```python
from build123d import *

# Parameters (mm, degrees)
F0_W           = 21.1
F0_H           = 25.1
F1_DEPTH       = 62.25
F2_W           = 21.1
F2_H           = 58.25
F3_DEPTH       = 25.4
F3_DEPTH_BACK  = 25.4
F4_W           = 3
F4_H           = 2
F5_DEPTH       = 25.4
F5_DEPTH_BACK  = 25.4
F6_W           = 25.1
F6_H           = 20
F7_DEPTH       = 11.1
F8_W           = 1
F8_H           = 3
F9_DEPTH       = 25.4
F9_DEPTH_BACK  = 25.4
F10_W          = 1
F10_H          = 3
F11_DEPTH      = 25.4
F11_DEPTH_BACK = 25.4


with BuildPart() as f1:
    # F0 (on Top) → F1 (new body)
    with BuildSketch(Plane.XY):
        with Locations((0.971473, 0)):
            Rectangle(F0_W, F0_H)
    extrude(amount=F1_DEPTH)

    # F2 (on face) → F3 (cut, two sides)
    with BuildSketch(Plane.YZ.offset(11.521473)) as f3_sk:
        with Locations((0, 31.125)):
            Rectangle(F2_W, F2_H)
    extrude(amount=-F3_DEPTH, mode=Mode.SUBTRACT)
    extrude(f3_sk.sketch, amount=-F3_DEPTH_BACK, mode=Mode.SUBTRACT)

    # F4 (on face) → F5 (cut, two sides)
    with BuildSketch(Plane.YZ.offset(11.521473)) as f5_sk:
        with Locations((0, 2)):
            Rectangle(F4_W, F4_H)
    extrude(amount=-F5_DEPTH, mode=Mode.SUBTRACT)
    extrude(f5_sk.sketch, amount=-F5_DEPTH_BACK, mode=Mode.SUBTRACT)

    # F6 (on face) → F7 (cut)
    with BuildSketch(Plane.YZ.offset(11.521473)):
        with Locations((0, 31.125)):
            Rectangle(F6_W, F6_H)
    extrude(amount=-F7_DEPTH, mode=Mode.SUBTRACT)

    # F8 (on face) → F9 (cut, two sides)
    with BuildSketch(Plane(origin=(0, 0, 0), x_dir=(1, 0, 0), z_dir=(0, 0, -1))) as f9_sk:
        with Locations((-9.078527, 0)):
            Rectangle(F8_W, F8_H)
    extrude(amount=-F9_DEPTH, mode=Mode.SUBTRACT)
    extrude(f9_sk.sketch, amount=-F9_DEPTH_BACK, mode=Mode.SUBTRACT)

    # F10 (on face) → F11 (cut, two sides)
    with BuildSketch(Plane(origin=(0, 0, 60.25), x_dir=(1, 0, 0), z_dir=(0, 0, -1))) as f11_sk:
        with Locations((-9.078527, 0)):
            Rectangle(F10_W, F10_H)
    extrude(amount=-F11_DEPTH, mode=Mode.SUBTRACT)
    extrude(f11_sk.sketch, amount=-F11_DEPTH_BACK, mode=Mode.SUBTRACT)


with BuildPart() as f12_1:
    # F12: copy of F1
    add(f1.part)


solid = f1.part
```
Can you work these out from the model? Positions are in its coordinate system, mm. A direction names the side the tool comes from. Coordinates: 2 decimals unless noted, no trailing zeros. Order: outer loops, then holes, each group sorted by start corner. A loop starts at its lowest first (then second) coordinate and runs counter-clockwise, first axis right, second up. Notation, with made-up numbers: (40, 46.5) - (48, 46.5) arc R32 ccw to (48, 83.5) - close; hole circle Ø10 at (-36, -6.75). An arc over 180 degrees is marked (long way). Answer in a Markdown table with one row per item.
1. Suppose I cut it at A-A (z = 24). Please give me the cut outline in (x, y).
Reply:
| item | result |
|---|---|
| outline | (-9.58, -12.55) - (0.42, -12.55) - (0.42, -10.55) - (-9.58, -10.55) - close; (-9.58, 10.55) - (0.42, 10.55) - (0.42, 12.55) - (-9.58, 12.55) - close |
2. For pin 1 (1.6 mm diameter, centred on x = 3.5, y = 11.5, fed in from -Z); pin 2 (12 mm diameter, centred on y = -7, z = 33.5, fed in from +X), each with a flat end and sliding along its axis, tell me the tip position at first contact or that it passes through.
Reply:
| item | result |
|---|---|
| pin 1 | stops at z = 0 |
| pin 2 | stops at x = 0.42 |
3. Suppose I cut it at C-C (x = 9). Please give me the cut outline in (y, z) (3 decimals), and give its area (3 significant figures).
Reply:
| item | result |
|---|---|
| outline | (-12.55, 0) - (12.55, 0) - (12.55, 21.125) - (10.55, 21.125) - (10.55, 2) - (1.5, 2) - (1.5, 1) - (-1.5, 1) - (-1.5, 2) - (-10.55, 2) - (-10.55, 21.125) - (-12.55, 21.125) - close; (-12.55, 41.125) - (-10.55, 41.125) - (-10.55, 60.25) - (10.55, 60.25) - (10.55, 41.125) - (12.55, 41.125) - (12.55, 62.25) - (-12.55, 62.25) - close |
| area | 250 mm^2 |
4. If I drill on line 1 along Y through (x, z) = (3, 48.5); line 2 along Z through (x, y) = (-5.25, 10.5); line 3 along Z through (x, y) = (9.5, -11.5) (3 decimals), over which ranges is the centre line in solid material (lowest first)?
Reply:
| item | result |
|---|---|
| line 1 | y = -12.55 to -10.55, 10.55 to 12.55 |
| line 2 | z = 0 to 2, 60.25 to 62.25 |
| line 3 | z = 0 to 21.125, 41.125 to 62.25 |
5. If we mould it in two halves opening along Z, with no side actions, what happens to faces 1 (the flat face through (1, 0, 62.25)), 2 (the flat face through (6, -12, 41.125)), 3 (the flat face through (1, 0, 0)), 4 (the flat face through (-9.579, 11, 38))? For each: pulls with the +Z half, pulls with the -Z half, needs draft (parallel to the pull), parting line crosses it, or undercut.
Reply:
| item | result |
|---|---|
| face 1 | pulls with the +Z half |
| face 2 | undercut |
| face 3 | pulls with the -Z half |
| face 4 | needs draft |
6. Suppose I cut it at D-D (x = -5). Please give me the cut outline in (y, z).
Reply:
| item | result |
|---|---|
| outline | (-12.55, 0) - (12.55, 0) - (12.55, 62.25) - (-12.55, 62.25) - close; hole (-10.55, 2) - (-1.5, 2) - (-1.5, 1) - (1.5, 1) - (1.5, 2) - (10.55, 2) - (10.55, 60.25) - (-10.55, 60.25) - close |
7. For faces 5 (the flat face through (6, 12, 41.125)), 6 (the flat face through (-8.579, 0, 61)), 7 (the flat face through (-1, -10.55, 31)), which set-ups out of +Z, -Z, +X, -X, +Y, -Y let a thin tool reach every point of the face, with its end or its side?
Reply:
| item | result |
|---|---|
| face 5 | +X, +Y, -Y |
| face 6 | +Z, -Z, -X |
| face 7 | +X, -X |
8. Suppose I cut it at B-B (y = -6.5). Please give me the cut outline in (x, z), and give its area (3 significant figures).
Reply:
| item | result |
|---|---|
| outline | (-9.58, 0) - (11.52, 0) - (11.52, 2) - (-9.58, 2) - close; (-9.58, 60.25) - (11.52, 60.25) - (11.52, 62.25) - (-9.58, 62.25) - close |
| area | 84.4 mm^2 |
